```python
from build123d import *

# Parameters (mm, degrees)
SKETCH_1_R      = 52.5
SKETCH_1_R_2    = 4
EXTRUDE_1_DEPTH = 3
FILLET_1_R      = 2


with BuildPart() as part:
    # 草图1 → 凸台-拉伸1 (new body)
    with BuildSketch(Plane.XY):
        Circle(SKETCH_1_R)
        Circle(SKETCH_1_R_2, mode=Mode.SUBTRACT)
        with BuildLine():
            Line((3, 47.405168495), (3, 9.539392014))
            ThreePointArc((3, 9.539392014), (7.071067812, 7.071067812), (9.539392014, 3))
            Line((9.539392014, 3), (47.405168495, 3))
            ThreePointArc((47.405168495, 3), (33.587572106, 33.587572106), (3, 47.405168495))
        make_face(mode=Mode.SUBTRACT)
        with BuildLine():
            Line((3, -9.539392014), (3, -47.405168495))
            ThreePointArc((3, -47.405168495), (33.587572106, -33.587572106), (47.405168495, -3))
            Line((47.405168495, -3), (9.539392014, -3))
            ThreePointArc((9.539392014, -3), (7.071067812, -7.071067812), (3, -9.539392014))
        make_face(mode=Mode.SUBTRACT)
        with BuildLine():
            Line((-3, 47.405168495), (-3, 9.539392014))
            ThreePointArc((-3, 9.539392014), (-7.071067812, 7.071067812), (-9.539392014, 3))
            Line((-9.539392014, 3), (-47.405168495, 3))
            ThreePointArc((-47.405168495, 3), (-33.587572106, 33.587572106), (-3, 47.405168495))
        make_face(mode=Mode.SUBTRACT)
        with BuildLine():
            Line((-47.405168495, -3), (-9.539392014, -3))
            ThreePointArc((-9.539392014, -3), (-7.071067812, -7.071067812), (-3, -9.539392014))
            Line((-3, -9.539392014), (-3, -47.405168495))
            ThreePointArc((-3, -47.405168495), (-33.587572106, -33.587572106), (-47.405168495, -3))
        make_face(mode=Mode.SUBTRACT)
    extrude(amount=EXTRUDE_1_DEPTH)

    # 圆角1
    fillet_1_edges = [part.edges().sort_by_distance(p)[0] for p in [
        (-3, 47.405168495, 1.5),
        (-47.405168495, 3, 1.5),
        (-9.539392014, 3, 1.5),
        (-3, 9.539392014, 1.5),
        (3, -47.405168495, 1.5),
        (47.405168495, -3, 1.5),
        (9.539392014, -3, 1.5),
        (3, -9.539392014, 1.5),
        (-47.405168495, -3, 1.5),
        (-3, -47.405168495, 1.5),
        (-3, -9.539392014, 1.5),
        (-9.539392014, -3, 1.5),
        (3, 9.539392014, 1.5),
        (9.539392014, 3, 1.5),
        (47.405168495, 3, 1.5),
        (3, 47.405168495, 1.5),
    ]]
    fillet(fillet_1_edges, radius=FILLET_1_R)


solid = part.part
```
Verification items for the finished model (mm, model axes). A direction names the side the tool comes from. Round coordinates to 2 decimals unless told otherwise and drop trailing zeros. Loops run counter-clockwise (first coordinate to the right, second up) from the corner with the lowest first, then second, coordinate; pieces in that order, holes last. Notation, with made-up numbers: (-6.75, 9.5) -> (38.25, 9.5) arc R17 ccw to (38.25, 23.5) -> close; hole circle Ø2 at (30.25, 46). An arc over 180 degrees is marked (long way). Answer as a JSON object with one key per item and string values.
Q1. Go/stop test with flat-tipped pins: P1, Ø1.5, axis at x = 31.5, z = 2, coming from the -Y side; P2, Ø0.9, axis at y = 33.5, z = 1.5, coming from the -X side; P3, Ø1.5, axis at y = -19.5, z = 1, coming from the +X side. Record where each tip stops, or that it passes through.
Data:
{"P1": "stops at y = -42.55", "P2": "stops at x = -40.79", "P3": "stops at x = 49.04"}
Q2. Draft check along X on faces 3 (the cylindrical face through (-0.867, -3.905, 1.479)), 4 (the cylindrical face through (50.076, 15.77, 1.479)), 5 (the flat face through (-1, -11, 3)). Enter one of: pulls with the +X half, pulls with the -X half, needs draft (parallel to the pull), parting line crosses it, or undercut.
Data:
{"face 3": "undercut", "face 4": "parting line crosses it", "face 5": "needs draft"}
Q3. Access from +Z, -Z, +X, -X, +Y, -Y to the whole of each face (thin tool, end or side, straight path). Record for faces 1 (the flat face through (-1, -11, 0)), 2 (the cylindrical face through (-7.036, 7.106, 1.479)).
Data:
{"face 1": "-Z, +X, -X, +Y, -Y", "face 2": "+Z, -Z"}
Q4. Section check D-D (x = -29). Record the boundary of the cut face in (y, z), then the cut area to 3 significant figures.
Data:
{"outline": "(-43.76, 0) -> (-37.62, 0) -> (-37.62, 3) -> (-43.76, 3) -> close; (-3, 0) -> (3, 0) -> (3, 3) -> (-3, 3) -> close; (37.62, 0) -> (43.76, 0) -> (43.76, 3) -> (37.62, 3) -> close", "area": "54.9 mm2"}
Q5. Section check A-A (y = 0). Record the boundary of the cut face in (x, z).
Data:
{"outline": "(-52.5, 0) -> (-4, 0) -> (-4, 3) -> (-52.5, 3) -> close; (4, 0) -> (52.5, 0) -> (52.5, 3) -> (4, 3) -> close"}
Q6. Section check C-C (z = 1.6). State how many separate pieces and enclosed holes the cut face has, then the cut area to 3 significant figures.
Data:
{"separate pieces": "1", "enclosed holes": "5", "area": "2,750 mm2"}
Q7. Scan lines: line 1 (Y direction, x = -6.5, z = 2.1); line 2 (Y direction, x = 18.5, z = 2.75); line 3 (Y direction, x = 0, z = 0.95). Record each from-to range of solid material in increasing order. Write a range as from..to.
Data:
{"line 1": "y = -52.1..-47.05, -7.6..7.6, 47.05..52.1", "line 2": "y = -49.13..-43.75, -3..3, 43.75..49.13", "line 3": "y = -52.5..-4, 4..52.5"}
